Read the model definition and answer for the solid it produces. Units are mm, in the model's axes. A direction names the side the tool comes from. Coordinates: 2 decimals unless noted, no trailing zeros. Write each loop counter-clockwise with the first axis right and the second up, starting at its lowest first coordinate (ties: lowest second). Pieces come first, ordered by that corner, then holes. Notation, with made-up numbers: (-18.5, 22.5) -> (32.5, 22.5) arc R17 cw to (32.5, 32.5) -> close; hole circle Ø10 at (47.25, 69). An arc over 180 degrees is marked (long way). One line per item, written item: value. Start each with the question number.
1. Find section A-A, the plane y = 3.25. Write down the section's boundary in (x, z), and give its area (3 significant figures).
2. Find section B-B, the plane x = 0. Write down the section's boundary in (y, z), and give its area (3 significant figures).
3. Find section C-C, the plane z = -15.5. State how many separate pieces and enclosed holes the cut face has, and give its area (3 significant figures).
4. Given P1, Ø1, axis at x = 0.5, z = -14, coming from the -Y side; P2, Ø12.5, axis at x = 8.5, z = 0.5, coming from the -Y side; P3, Ø5, axis at x = -11.5, y = 3, coming from the -Z side, each flat-ended and moving along its own axis, determine where each tip first touches the part or whether it passes through.
5. For faces 4 (the flat face through (0, 8.3, -16)), 5 (the flat face through (9, 8.3, 9)), 6 (the cylindrical face through (2.43, 6.9, -16.07)), determine the directions among +Z, -Z, +X, -X, +Y, -Y from which every point of the face is accessible in a straight line to the end or side of a thin tool.
6. Find section D-D, the plane z = 0. Write down the section's boundary in (x, y).
7. For a pull along X with two mould halves and no side action, classify faces 1 (the flat face through (9, 10.3, 9)), 2 (the cylindrical face through (-17.235, 5.078, 15.272)), 3 (the flat face through (-21.15, 9, 0)) as pulls with the +X half, pulls with the -X half, needs draft (parallel to the pull), parting line crosses it, or undercut.
8. Consider line 1 along X through (y, z) = (5.5, 15.5); line 2 along X through (y, z) = (7.5, -13). Determine where each line is inside the solid, lowest interval first.
```python
from build123d import *
from build123d.topology import SkipClean

# Parameters (mm, degrees)
SKETCH1_R               = 3.25
BOSS_EXTRUDE1_DEPTH     = 10.3
SKETCH2_W               = 42.3
SKETCH2_H               = 42.3
SKETCH2_R               = 11.25
BOSS_EXTRUDE2_DEPTH     = 2
CUT_EXTRUDE1_DEPTH      = 32.634395837
SKETCH4_R               = 1.75
CUT_EXTRUDE2_DEPTH      = 32.634395837
MIRROR6_COPY_1_SKETCH_R = 1.75
MIRROR6_COPY_1_DEPTH    = 32.634395837
BOSS_EXTRUDE3_DEPTH     = 2
CUT_EXTRUDE3_DEPTH      = 2
FILLET1_R               = 2


with BuildPart() as part:
    # Sketch1 → Boss-Extrude1 (new body)
    with BuildSketch(Plane(origin=(0, 0, 0), x_dir=(1, 0, 0), z_dir=(0, 1, 0))):
        with Locations(Location((-15.5, 15.5, 0), (0, 0, 90))):
            Circle(SKETCH1_R)
    extrude(amount=BOSS_EXTRUDE1_DEPTH)


with BuildPart() as body_2:
    # Mirror2: mirrored copy
    add(part.part.mirror(Plane(origin=(0, 0, 0), x_dir=(0, 0, 1), z_dir=(1, 0, 0))))


with BuildPart() as body_3:
    # Mirror3: mirrored copy
    add(part.part.mirror(Plane.XY))


with BuildPart() as body_4:
    # Mirror3 2: mirrored copy
    add(body_2.part.mirror(Plane.XY))


with BuildPart() as part_1:
    add(part.part)

    add(body_2.part)  # Boss-Extrude2 merges body 2

    add(body_3.part)  # Boss-Extrude2 merges body 3

    add(body_4.part)  # Boss-Extrude2 merges body 4
    # Sketch2 → Boss-Extrude2 (add)
    with BuildSketch(Plane(origin=(0, 10.3, 0), x_dir=(1, 0, 0), z_dir=(0, 1, 0))):
        Rectangle(SKETCH2_W, SKETCH2_H)
        with Locations(Location((0, 0, 0), (0, 0, 270))):
            Circle(SKETCH2_R, mode=Mode.SUBTRACT)
    extrude(amount=-BOSS_EXTRUDE2_DEPTH)

    # Sketch3 → Cut-Extrude1 (cut, through all)
    with BuildSketch(Plane(origin=(0, 10.3, 0), x_dir=(1, 0, 0), z_dir=(0, 1, 0))):
        Polygon((-16.963055506, 21.15), (-21.15, 16.963055506), (-21.15, 21.15), align=None)
        Polygon((16.963055506, -21.15), (21.15, -16.963055506), (21.15, -21.15), align=None)
    cut_extrude1 = extrude(amount=-CUT_EXTRUDE1_DEPTH, mode=Mode.SUBTRACT)

    # Mirror4: Cut-Extrude1 across plane
    add(cut_extrude1.mirror(Plane.XY), mode=Mode.SUBTRACT)

    # Sketch4 → Cut-Extrude2 (cut, through all)
    with BuildSketch(Plane.XZ):
        with Locations(Location((15.5, -15.5, 0), (0, 0, 270))):
            Circle(SKETCH4_R)
    cut_extrude2 = extrude(amount=-CUT_EXTRUDE2_DEPTH, mode=Mode.SUBTRACT)

    # Mirror5: Cut-Extrude2 across plane
    add(cut_extrude2.mirror(Plane(origin=(0, 0, 0), x_dir=(0, 0, 1), z_dir=(1, 0, 0))), mode=Mode.SUBTRACT)

    # Mirror6: Cut-Extrude2 across plane
    add(cut_extrude2.mirror(Plane.XY), mode=Mode.SUBTRACT)

    # Mirror6 copy 1 sketch → Mirror6 copy 1 (cut, through all)
    with BuildSketch(Plane(origin=(0, 0, 0), x_dir=(-1, 0, 0), z_dir=(0, -1, 0))):
        with Locations(Location((15.5, -15.5, 0), (0, 0, 270))):
            Circle(MIRROR6_COPY_1_SKETCH_R)
    extrude(amount=-MIRROR6_COPY_1_DEPTH, mode=Mode.SUBTRACT)

    # Sketch6 → Boss-Extrude3 (add)
    with SkipClean():  # the faces are left unmerged after this step: merging them gives an invalid solid
        with BuildSketch(Plane.XZ.offset(-8.3)):
            with BuildLine():
                Line((-3, -21.15), (-3, -10.842624221))
                ThreePointArc((-3, -10.842624221), (0, -11.25), (3, -10.842624221))
                Line((3, -10.842624221), (3, -21.15))
                Line((3, -21.15), (-3, -21.15))
            make_face()
        extrude(amount=BOSS_EXTRUDE3_DEPTH)

    # Sketch7 → Cut-Extrude3 (cut)
    with SkipClean():  # the faces are left unmerged after this step: merging them gives an invalid solid
        with BuildSketch(Plane(origin=(0, 10.3, 0), x_dir=(1, 0, 0), z_dir=(0, 1, 0))):
            with BuildLine():
                Line((-1, 11.25), (-1, 21.15))
                ThreePointArc((-1, 21.15), (0, 22.15), (1, 21.15))
                Line((1, 21.15), (1, 11.25))
                ThreePointArc((1, 11.25), (0, 10.25), (-1, 11.25))
            make_face()
        extrude(amount=-CUT_EXTRUDE3_DEPTH, mode=Mode.SUBTRACT)

    # Fillet1
    fillet1_edges = [part_1.edges().sort_by_distance(p)[0] for p in [
        (3, 6.3, -15.996312111),
        (-3, 6.3, -15.996312111),
    ]]
    fillet(fillet1_edges, radius=FILLET1_R - 0.0001)  # a hair under: the kernel refuses the full size


solid = part_1.part
```
Answer block:
1. outline: circle Ø6.5 at (-15.5, -15.5); circle Ø6.5 at (-15.5, 15.5); circle Ø6.5 at (15.5, -15.5); circle Ø6.5 at (15.5, 15.5); hole circle Ø3.5 at (-15.5, -15.5); hole circle Ø3.5 at (-15.5, 15.5); hole circle Ø3.5 at (15.5, -15.5); hole circle Ø3.5 at (15.5, 15.5)
1. area: 94.2 mm2
2. outline: (6.3, -21.15) -> (8.3, -21.15) -> (8.3, -11.25) -> (6.3, -11.25) -> close; (8.3, 11.25) -> (10.3, 11.25) -> (10.3, 21.15) -> (8.3, 21.15) -> close
2. area: 39.6 mm2
3. separate pieces: 3
3. enclosed holes: 0
3. area: 127 mm2
4. P1: stops at y = 6.3
4. P2: stops at y = 8.3
4. P3: stops at z = -18.38
5. face 4: -Z, +Y
5. face 5: -Y
5. face 6: +Z, -Z, -Y
6. outline: (-21.15, 8.3) -> (-11.25, 8.3) -> (-11.25, 10.3) -> (-21.15, 10.3) -> close; (11.25, 8.3) -> (21.15, 8.3) -> (21.15, 10.3) -> (11.25, 10.3) -> close
7. face 1: needs draft
7. face 2: undercut
7. face 3: pulls with the -X half
8. line 1: x = -18.75 to -17.25, -13.75 to -12.25, 12.25 to 13.75, 17.25 to 18.75
8. line 2: x = -17.58 to -13.42, -2.83 to 2.83, 13.42 to 17.58
